For this review, take the finished solid that the model builds, in its own axes (mm). A direction names the side the tool comes from. Coordinates: 2 decimals unless noted, no trailing zeros. Order: outer loops, then holes, each group sorted by start corner. A loop starts at its lowest first (then second) coordinate and runs counter-clockwise, first axis right, second up. Notation, with made-up numbers: (10, 48) -> (31, 48) arc R22 cw to (31, 87) -> close; hole circle Ø7 at (-35, 2.5). An arc over 180 degrees is marked (long way). Return JSON: item names as keys, results as strings. Group by question number.
Item 1: Insertion check: pin 1 (4.5 mm diameter, centred on x = -23.57, z = -23.57, fed in from -Y); pin 2 (5 mm diameter, centred on x = -25.5, y = 45.5, fed in from -Z); pin 3 (1.4 mm diameter, centred on x = 26, y = 28, fed in from +Z); pin 4 (1.4 mm diameter, centred on y = 61.5, z = -26, fed in from +X). Each pin has a flat end and moves straight along its axis. Give the tip position at first contact, or say it passes through.
Item 2: Machinability: for faces 1 (the flat face through (-26, 54, 17.57)), 2 (the cylindrical face through (19.281, 54.329, -19.374)), 3 (the flat face through (26, 54, 17.57)), which of the approach directions +Z, -Z, +X, -X, +Y, -Y give a long, thin tool a straight path to every point of the face, cutting with its end or side? Answer none if there is none.
Item 3: For line 1 along Y through (x, z) = (7, 16); line 2 along X through (y, z) = (-1, -23); line 3 along Z through (x, y) = (-25, 13), list the stretches that pass through material, from the lowest coordinate up.
Item 4: Draft analysis for pull direction X (two halves, no side actions). For faces 4 (the flat face through (-17.57, 54, 26)), 5 (the flat face through (4, -6.4, 0)), 6 (the cylindrical face through (-22.39, -2.37, 21.31)), state which applies: +X half, -X half, draft (parallel to the pull), parting line (faces both ways), or undercut.
Item 5: Take a section at C-C (y = -10.5). Write out the cut boundary in (x, z) (3 decimals), then the cut area to 3 significant figures.
```python
from build123d import *

# Parameters (mm, degrees)
SKETCH_R     = 2.55
PAD_DEPTH    = 4.8
SKETCH001_R  = 19.05
PAD001_DEPTH = 1.6
SKETCH002_R  = 3.175
PAD002_DEPTH = 19
PAD003_DEPTH = 4.8
PAD004_DEPTH = 95.8
PAD005_DEPTH = 9.6


with BuildPart() as part:
    # Sketch → Pad (new body)
    with BuildSketch(Plane.XZ):
        with BuildLine():
            ThreePointArc((-23.569992, 28.200011), (-26.843905, 26.843912), (-28.200003, 23.57))
            Line((-28.200003, 23.57), (-28.200003, -23.569985))
            ThreePointArc((-28.200003, -23.569985), (-26.84391, -26.843907), (-23.569992, -28.200011))
            Line((-23.569992, -28.200011), (23.569992, -28.200011))
            ThreePointArc((23.569992, -28.200011), (26.843903, -26.843907), (28.199997, -23.569992))
            Line((28.199997, 23.569992), (28.199997, -23.569992))
            ThreePointArc((28.199997, 23.569992), (26.843903, 26.843907), (23.569992, 28.200011))
            Line((-23.569992, 28.200011), (23.569992, 28.200011))
        make_face()
        with Locations((-23.569992, 23.57)):
            Circle(SKETCH_R, mode=Mode.SUBTRACT)
        with Locations((23.569985, 23.57)):
            Circle(SKETCH_R, mode=Mode.SUBTRACT)
        with Locations((23.569985, -23.57)):
            Circle(SKETCH_R, mode=Mode.SUBTRACT)
        with Locations((-23.569992, -23.57)):
            Circle(SKETCH_R, mode=Mode.SUBTRACT)
    extrude(amount=PAD_DEPTH)

    # Sketch001 → Pad001 (new body)
    with BuildSketch(Plane.XZ.offset(4.8)):
        Circle(SKETCH001_R)
    extrude(amount=PAD001_DEPTH)

    # Sketch002 → Pad002 (new body)
    with BuildSketch(Plane.XZ.offset(6.4)):
        Circle(SKETCH002_R)
    extrude(amount=PAD002_DEPTH)

    # Sketch003 → Pad003 (new body)
    with BuildSketch(Plane(origin=(0, 0, 0), x_dir=(1, 0, 0), z_dir=(0, 1, 0))):
        with BuildLine():
            ThreePointArc((-23.569999, 17.57), (-19.327359, 19.32736), (-17.57, 23.570001))
            Line((-17.57, 23.570001), (-17.57, 28.2))
            Line((-17.57, 28.2), (17.57, 28.2))
            Line((17.57, 28.2), (17.57, 23.56997))
            ThreePointArc((17.57, 23.56997), (19.32737, 19.327349), (23.57, 17.57))
            Line((23.57, 17.57), (28.2, 17.57))
            Line((28.2, 17.57), (28.2, -17.57))
            Line((28.2, -17.57), (23.570008, -17.57))
            ThreePointArc((23.570008, -17.57), (19.327365, -19.327354), (17.57, -23.569992))
            Line((17.57, -28.2), (17.57, -23.569992))
            Line((-17.57, -28.2), (17.57, -28.2))
            Line((-17.57, -23.57), (-17.57, -28.2))
            ThreePointArc((-17.57, -23.57), (-19.327359, -19.327359), (-23.57, -17.57))
            Line((-28.2, -17.57), (-23.57, -17.57))
            Line((-28.2, 17.57), (-28.2, -17.57))
            Line((-23.569999, 17.57), (-28.2, 17.57))
        make_face()
    extrude(amount=PAD003_DEPTH)

    # Sketch004 → Pad004 (new body)
    with BuildSketch(Plane(origin=(0, 4.8, 0), x_dir=(1, 0, 0), z_dir=(0, 1, 0))):
        with BuildLine():
            ThreePointArc((-23.569999, 17.57), (-19.327359, 19.32736), (-17.57, 23.570001))
            Line((-17.57, 23.570001), (-17.57, 28.2))
            Line((-17.57, 28.2), (17.57, 28.2))
            Line((17.57, 28.2), (17.57, 23.56997))
            ThreePointArc((17.57, 23.56997), (19.32737, 19.327349), (23.57, 17.57))
            Line((23.57, 17.57), (28.2, 17.57))
            Line((28.2, 17.57), (28.2, -17.57))
            Line((28.2, -17.57), (23.570008, -17.57))
            ThreePointArc((23.570008, -17.57), (19.327365, -19.327354), (17.57, -23.569992))
            Line((17.57, -28.2), (17.57, -23.569992))
            Line((-17.57, -28.2), (17.57, -28.2))
            Line((-17.57, -23.57), (-17.57, -28.2))
            ThreePointArc((-17.57, -23.57), (-19.327359, -19.327359), (-23.57, -17.57))
            Line((-28.2, -17.57), (-23.57, -17.57))
            Line((-28.2, 17.57), (-28.2, -17.57))
            Line((-23.569999, 17.57), (-28.2, 17.57))
        make_face()
    extrude(amount=PAD004_DEPTH)

    # Sketch005 → Pad005 (new body)
    with BuildSketch(Plane(origin=(0, 100.6, 0), x_dir=(1, 0, 0), z_dir=(0, 1, 0))):
        with BuildLine():
            ThreePointArc((-23.569999, 17.57), (-19.327359, 19.32736), (-17.57, 23.570001))
            Line((-17.57, 23.570001), (-17.57, 28.2))
            Line((-17.57, 28.2), (17.57, 28.2))
            Line((17.57, 28.2), (17.57, 23.56997))
            ThreePointArc((17.57, 23.56997), (19.32737, 19.327349), (23.57, 17.57))
            Line((23.57, 17.57), (28.2, 17.57))
            Line((28.2, 17.57), (28.2, -17.57))
            Line((28.2, -17.57), (23.570008, -17.57))
            ThreePointArc((23.570008, -17.57), (19.327365, -19.327354), (17.57, -23.569992))
            Line((17.57, -28.2), (17.57, -23.569992))
            Line((-17.57, -28.2), (17.57, -28.2))
            Line((-17.57, -23.57), (-17.57, -28.2))
            ThreePointArc((-17.57, -23.57), (-19.327359, -19.327359), (-23.57, -17.57))
            Line((-28.2, -17.57), (-23.57, -17.57))
            Line((-28.2, 17.57), (-28.2, -17.57))
            Line((-23.569999, 17.57), (-28.2, 17.57))
        make_face()
    extrude(amount=PAD005_DEPTH)


solid = part.part
```
Findings below:
{
 "1": {"pin 1": "passes through", "pin 2": "stops at z = -17.6", "pin 3": "stops at z = 17.57", "pin 4": "stops at x = 17.57"},
 "2": {"face 1": "+Z, -X, +Y", "face 2": "-Z, +X, +Y", "face 3": "+Z, +X, +Y"},
 "3": {"line 1": "y = -6.4 to 110.2", "line 2": "x = -28.2 to -26.06, -21.08 to 21.08, 26.06 to 28.2", "line 3": "z = -17.57 to 17.57"},
 "4": {"face 4": "-X half", "face 5": "draft", "face 6": "undercut"},
 "5": {"outline": "circle Ø6.35 at (0, 0)", "area": "31.7 mm2"}
}
